Source: CAD feature listing. Evaluate the final solid. Frame: model axes, mm. A direction names the side the tool comes from. Give positions to 0.01 mm unless a question says otherwise; leave off trailing zeros. Order: outer loops, then holes, each group sorted by start corner. A loop starts at its lowest first (then second) coordinate and runs counter-clockwise, first axis right, second up.
Autodesk Inventor part; units mm, degrees
ref_plane "YZ Plane" through (0, 0, 0) normal (1, 0, 0) x (0, 1, 0)
ref_plane "XZ Plane" through (0, 0, 0) normal (0, 1, 0) x (-1, 0, 0)
ref_plane "XY Plane" through (0, 0, 0) normal (0, 0, 1) x (1, 0, 0)
sketch "Sketch1" plane through (0, 0, 0) normal (0, 0, 1) x (1, 0, 0)
  line L0 (-60, 0) -> (60, 0)
  line L1 (70, -50) -> (70, -65)
  line L2 (70, -65) -> (-70, -65)
  line L3 (-70, -65) -> (-70, -50)
  line L4 (-70, -50) -> (70, -65) construction
  line L5 (-70, -50) -> (-33.1662, -50)
  line L6 (33.1662, -50) -> (70, -50)
  arc A0 (-60, 0) -> (-33.1662, -50) centre (0, 0) ccw
  arc A1 (33.1662, -50) -> (60, 0) centre (0, 0) ccw
  line L7 (70, -50) -> (24.1881, -54.9084) construction
  line L8 (0, -57.5) -> (-70, -65) construction
  dimension "d1" = 15
  dimension "d2" = 140
  dimension "d3" = 0
  dimension "d4" = 65
extrude "Extrusion1" add sketch "Sketch1" along normal mid plane 80
shell "Shell1" thickness 1 removed faces 1 at (-20, 0, 13.3333)
sketch "Sketch2" plane through (0, 0, 40) normal (0, 0, 1) x (1, 0, 0)
  circle A0 centre (0, 0) radius 45
  dimension "d8" = 90
extrude "Extrusion2" cut sketch "Sketch2" against normal blind 2
sketch "Sketch3" plane through (-69, -64, -39) normal (0, 0, 1) x (1, 0, 0)
  circle A0 centre (69, 64) radius 15
  dimension "d11" = 30
extrude "Extrusion3" cut sketch "Sketch3" against normal blind 2
sketch "Sketch4" plane through (0, 0, 0) normal (0, 0, 1) x (1, 0, 0)
  line L0 (60, 0) -> (45, 0)
  line L1 (59.4, 0) -> (75, 0)
  line L2 (75, 0) -> (75, -4)
  line L3 (75, -4) -> (59.4, -4)
  line L4 (59.4, -4) -> (59.4, 0)
  line L5 (-70, -65) -> (70, -65)
  line L6 (0, 14.3485) -> (0, -121.7011) construction
  line L7 (-60, 0) -> (-45, 0)
  line L8 (-59.4, 0) -> (-75, 0)
  line L9 (-75, 0) -> (-75, -4)
  line L10 (-75, -4) -> (-59.4, -4)
  line L11 (-59.4, -4) -> (-59.4, 0)
  point P0 (0, 0)
  dimension "d14" = 65
  dimension "d15" = 4
  dimension "d16" = 15.6
  dimension "d17" = 75
extrude "Extrusion4" add sketch "Sketch4" along normal mid plane 80
sketch "Sketch5" plane through (59.8665, -4, -40) normal (0, -1, 0) x (1, 0, 0)
  circle A0 centre (7.6335, 10) radius 2.05
  line L0 (15.1335, 0) -> (0, 0)
  line L1 (15.1335, 80) -> (15.1335, 0)
  circle A1 centre (7.6335, 30) radius 2.05
  circle A2 centre (7.6335, 50) radius 2.05
  circle A3 centre (7.6335, 70) radius 2.05
  circle A4 centre (-127.3665, 10) radius 2.05
  circle A5 centre (-127.3665, 30) radius 2.05
  circle A6 centre (-127.3665, 50) radius 2.05
  circle A7 centre (-127.3665, 70) radius 2.05
  point P0 (-59.8665, 40)
  point P1 (15.1335, 20)
  point P2 (15.1335, 40)
  point P3 (15.1335, 60)
  point P4 (-119.8665, 0)
  point P5 (-119.8665, 20)
  point P6 (-119.8665, 40)
  point P7 (-119.8665, 60)
  dimension "d20" = 4.1
  dimension "d21" = 10
  dimension "d22" = 7.5
  dimension "d25" = 20
  dimension "d28" = 135
extrude "Extrusion5" cut sketch "Sketch5" against normal blind 80
properties part number "Carcaça Inferior do Motor Industiral" material "Aluminum 6061"
1) Reachability of faces 4 (the face through (66, -2, 31.4)), 5 (the face through (-69, -58, -1)), 6 (the face through (-68, -4, -1)) from +Z, -Z, +X, -X, +Y, -Y: full face, straight path, thin tool, end or side. Return the list, or none.
Checks:
face 4: +Y
face 5: none
face 6: +Z, -Z, -X
2) Pull-direction query (Z, two-part tool) for faces 1 (the face through (-1, -32, -40)), 2 (the face through (51.36, -29.04, -0.55)), 3 (the face through (68, -4, -1)); classes: +Z half, -Z half, draft (parallel to the pull), parting line (faces both ways), or undercut.
Checks:
face 1: -Z half
face 2: undercut
face 3: draft
3) Ray query, L1, parallel to Y at x = -64.5, z = 37.5; L2, parallel to X at y = -55, z = 8; L3, parallel to Z at x = 67.5, y = -2.35. Return the intervals inside material, ascending.
Checks:
L1: y = -65 to -64, -51 to -50, -4 to 0
L2: x = -70 to -69, 69 to 70
L3: z = -40 to -32.05, -27.95 to -12.05, -7.95 to 7.95, 12.05 to 27.95, 32.05 to 40
4) Section query B-B on z = -30. Output: boundary loops of the cut face in (x, y).
Checks:
outline: (-75, -4) - (-69.55, -4) - (-69.55, 0) - (-75, 0) - close; (-70, -65) - (70, -65) - (70, -50) - (33.17, -50) arc R60 ccw to (59.87, -4) - (65.45, -4) - (65.45, 0) - (59, 0) arc R59 cw to (29.66, -51) - (69, -51) - (69, -64) - (-69, -64) - (-69, -51) - (-29.66, -51) arc R59 cw to (-59, 0) - (-65.45, 0) - (-65.45, -4) - (-59.87, -4) arc R60 ccw to (-33.17, -50) - (-70, -50) - close; (69.55, -4) - (75, -4) - (75, 0) - (69.55, 0) - close
5) First-contact query: pin 1 Ø16.5 at (y, z) = (-58.5, -8) entering from +X; pin 2 Ø16.5 at (y, z) = (-56, -11.5) entering from -X; pin 3 Ø6 at (y, z) = (-43.5, 12.5) entering from +X. Flat tips, straight axial feed; report the tip coordinate or a pass-through.
Checks:
pin 1: stops at x = 70
pin 2: stops at x = -70
pin 3: stops at x = 44.27
6) Section query A-A on x = 62. Output: boundary loops of the cut face in (y, z), and give its area (3 significant figures).
Checks:
outline: (-65, -40) - (-50, -40) - (-50, 40) - (-65, 40) - close; (-4, -40) - (0, -40) - (0, 40) - (-4, 40) - close; hole (-64, -39) - (-51, -39) - (-51, 39) - (-64, 39) - close
area: 506 mm2
